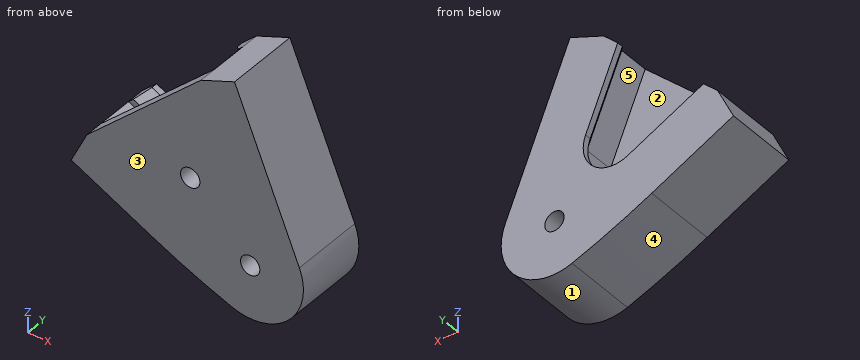
from build123d import *
from build123d.topology import SkipClean

# Parameters (mm, degrees)
SKETCH1_R           = 1.6
BOSS_EXTRUDE1_DEPTH = 6
BOSS_EXTRUDE3_START = 3
SKETCH7_R           = 1.6
BOSS_EXTRUDE3_DEPTH = 3
SKETCH8_R           = 1.6
BOSS_EXTRUDE4_DEPTH = 3
CHAMFER1_SIZE       = 2


with BuildPart() as part:
    # Sketch1 → Boss-Extrude1 (new body)
    with BuildSketch(Plane(origin=(0, 0, 0), x_dir=(1, 0, 0), z_dir=(0, 1, 0))):
        with BuildLine():
            Line((40.930223616, 79.991972891), (54.42997891, 86.530826536))
            ThreePointArc((54.42997891, 86.530826536), (63.577181794, 85.122585909), (65.51014962, 76.071724202))
            Line((65.51014962, 76.071724202), (59.760023318, 62.21762562))
            Line((59.760023318, 62.21762562), (65.30166275, 59.917575099))
            Line((65.30166275, 59.917575099), (76.011513854, 85.721414039))
            ThreePointArc((76.011513854, 85.721414039), (74.278699447, 95.141487045), (64.97108226, 97.401726747))
            ThreePointArc((64.97108226, 97.401726747), (58.314802122, 94.853700296), (51.814437452, 91.930728654))
            Line((51.814437452, 91.930728654), (38.314682158, 85.391875009))
            Line((38.314682158, 85.391875009), (40.930223616, 79.991972891))
        make_face()
        with Locations(Location((67.882250994, 89.09545443, 0), (0, 0, 270))):
            Circle(SKETCH1_R, mode=Mode.SUBTRACT)
    extrude(amount=BOSS_EXTRUDE1_DEPTH)

    # Sketch7 → Boss-Extrude3 (add)
    with SkipClean():  # the faces are left unmerged after this step: merging them gives an invalid solid
        with BuildSketch(Plane.XZ.offset(BOSS_EXTRUDE3_START)):
            with BuildLine():
                Line((76.011513854, -85.721414039), (65.30166275, -59.917575099))
                Line((65.30166275, -59.917575099), (59.760023318, -62.21762562))
                Line((59.760023318, -62.21762562), (40.930223616, -79.991972891))
                Line((40.930223616, -79.991972891), (38.314682158, -85.391875009))
                Line((38.314682158, -85.391875009), (51.814437452, -91.930728654))
                ThreePointArc((51.814437452, -91.930728654), (58.314802122, -94.853700296), (64.97108226, -97.401726747))
                ThreePointArc((64.97108226, -97.401726747), (74.278699447, -95.141487045), (76.011513854, -85.721414039))
            make_face()
            with Locations(Location((67.882250994, -89.09545443, 0), (0, 0, 270))):
                Circle(SKETCH7_R, mode=Mode.SUBTRACT)
            with Locations(Location((57.982756057, -79.195959493, 0), (0, 0, 270))):
                Circle(SKETCH7_R, mode=Mode.SUBTRACT)
        extrude(amount=-BOSS_EXTRUDE3_DEPTH)

    # Sketch8 → Boss-Extrude4 (add)
    with BuildSketch(Plane(origin=(0, 6, 0), x_dir=(1, 0, 0), z_dir=(0, 1, 0))):
        with BuildLine():
            Line((38.314682158, 85.391875009), (40.930223616, 79.991972891))
            Line((40.930223616, 79.991972891), (43.264016412, 77.788994406))
            Line((43.264016412, 77.788994406), (55.737749639, 83.830875477))
            ThreePointArc((55.737749639, 83.830875477), (61.517883977, 82.941005633), (62.739329904, 77.221749462))
            Line((62.739329904, 77.221749462), (57.426230521, 64.420604105))
            Line((57.426230521, 64.420604105), (59.760023318, 62.21762562))
            Line((59.760023318, 62.21762562), (65.30166275, 59.917575099))
            Line((65.30166275, 59.917575099), (76.011513854, 85.721414039))
            ThreePointArc((76.011513854, 85.721414039), (74.278699447, 95.141487045), (64.97108226, 97.401726747))
            ThreePointArc((64.97108226, 97.401726747), (58.314802122, 94.853700296), (51.814437452, 91.930728654))
            Line((51.814437452, 91.930728654), (38.314682158, 85.391875009))
        make_face()
        with Locations(Location((67.882250994, 89.09545443, 0), (0, 0, 90))):
            Circle(SKETCH8_R, mode=Mode.SUBTRACT)
    extrude(amount=BOSS_EXTRUDE4_DEPTH)

    # Chamfer1
    chamfer1_edges = [part.edges().sort_by_distance(p)[0] for p in [
        (49.500883026, 6, -80.809934942),
        (61.517883977, 6, -82.941005633),
        (60.082780212, 6, -70.821176784),
    ]]
    chamfer(chamfer1_edges, length=CHAMFER1_SIZE)


solid = part.part
Verification items for the finished model (mm, model axes). Face numbers are marked on the shaded views. A direction names the side the tool comes from. Round coordinates to 2 decimals unless told otherwise and drop trailing zeros. Loops run counter-clockwise (first coordinate to the right, second up) from the corner with the lowest first, then second, coordinate; pieces in that order, holes last. Notation, with made-up numbers: (78.5, -12.75) - (115.5, -12.75) arc R16 cw to (115.5, 18.25) - close; hole circle Ø2 at (-30.75, 16). An arc over 180 degrees is marked (long way). Use one line per item in the form item = value.
1. Section check C-C on x = 50. Record the cut outline in (y, z).
A:
outline = (-3, -91.05) - (9, -91.05) - (9, -81.05) - (8, -81.05) - (6, -83.27) - (6, -84.39) - (0, -84.39) - (0, -71.43) - (-3, -71.43) - close
2. Section check D-D on y = -2. Record the cut outline in (x, z), and give its area (3 significant figures).
A:
outline = (38.31, -85.39) - (51.81, -91.93) arc R125.1 ccw to (64.97, -97.4) arc R8.8 ccw to (76.01, -85.72) - (65.3, -59.92) - (59.76, -62.22) - (40.93, -79.99) - close; hole circle Ø3.2 at (57.98, -79.2); hole circle Ø3.2 at (67.88, -89.1)
area = 826 mm²
3. Draft check along Z on the marked faces 1, 2 and 3. Enter one of: pulls with the +Z half, pulls with the -Z half, needs draft (parallel to the pull), parting line crosses it, or undercut.
A:
face_1 = parting line crosses it
face_2 = undercut
face_3 = needs draft
4. Scan lines: probe 1 along Y at (x, z) = (63, -85); probe 2 along X at (y, z) = (0.75, -85); probe 3 along X at (y, z) = (5.25, -90). Record each from-to range of solid material in increasing order.
A:
probe_1 = -3 to 0, 6 to 9
probe_2 = 38.5 to 51.27, 63.7 to 75.71
probe_3 = 47.83 to 66.56, 69.2 to 76.64
5. Section check B-B on z = -67.5. Record the cut outline in (x, y).
A:
outline = (54.16, -3) - (68.45, -3) - (68.45, 9) - (58.7, 9) - (58.7, 8) - (60.87, 6) - (61.95, 6) - (61.95, 0) - (54.16, 0) - close
6. Access from +Z, -Z, +X, -X, +Y, -Y to the whole of each face (thin tool, end or side, straight path). Record for the marked faces 4 and 5.
A:
face_4 = -Z, -X, +Y, -Y
face_5 = -X
7. Gauge pin test, flat ends, axial feed: pin 1 Ø2 at (y, z) = (5, -76.5) entering from +X; pin 2 Ø1 at (x, y) = (54.5, 1.5) entering from -Z; pin 3 Ø1 at (x, y) = (66.5, 7.5) entering from -Z. Record the tip position at first contact, or that the pin passes through.
A:
pin_1 = 72.6
pin_2 = -93.42
pin_3 = -97.85
8. Section check A-A on y = 1.5. Record the cut outline in (x, z).
A:
outline = (38.31, -85.39) - (51.81, -91.93) arc R125.1 ccw to (64.97, -97.4) arc R8.8 ccw to (76.01, -85.72) - (65.3, -59.92) - (59.76, -62.22) - (65.51, -76.07) arc R8.15 cw to (54.43, -86.53) - (40.93, -79.99) - close; hole circle Ø3.2 at (67.88, -89.1)
